The listing builds one solid part. Answer for the finished solid, in the listing's coordinates (mm). Face numbers are marked on the shaded views. A direction names the side the tool comes from. Round coordinates to 2 decimals unless told otherwise and drop trailing zeros. Write each loop counter-clockwise with the first axis right and the second up, starting at its lowest first coordinate (ties: lowest second). Pieces come first, ordered by that corner, then holes. Notation, with made-up numbers: (35.25, 72.25) - (53.25, 72.25) arc R3 ccw to (53.25, 76.25) - close; hole circle Ø2 at (-32.75, 35). An arc over 180 degrees is marked (long way). Use a Markdown table: item, result. Add a question column.
1) A cutting plane is placed at B-B (y = -5). Give the vertices of the cut face in (x, z), then the cut area to 3 significant figures.
2) A tool of negligible diameter and unlimited length cuts with its end or side. For the marked faces 1, 2, 3 and 4, from which of +Z, -Z, +X, -X, +Y, -Y can it reach the whole face along a straight path? Write none if from no direction.
3) A cutting plane is placed at A-A (x = 3). Give the vertices of the cut face in (y, z).
4) Each of these flat-tipped pins is pushed along its axis until it touches: P1, Ø5, axis at x = -3.68, z = 13.02, coming from the -Y side; P2, Ø5, axis at y = -3, z = 27.5, coming from the +X side; P3, Ø3, axis at y = -5, z = 31, coming from the -X side; P4, Ø4, axis at x = -5, z = 22.5, coming from the +Y side. Where does it stop, or does it pass through?
5) Find the intervals of material crossed by probe 1 along Z at (x, y) = (-2.5, 1.5); probe 2 along Z at (x, y) = (-1.5, 7.5); probe 3 along X at (y, z) = (4.75, 11), in increasing order. Write a range as from..to.
6) A cutting plane is placed at D-D (y = 0.5). Give the vertices of the cut face in (x, z), then the cut area to 3 significant figures.
7) Determine the mould class of the marked faces 5, 6 and 7 for opening direction Z: +Z half, -Z half, draft (parallel to the pull), parting line (faces both ways), or undercut.
8) A cutting plane is placed at C-C (x = 0). Give the vertices of the cut face in (y, z).
```python
from build123d import *

# Parameters (mm, degrees)
F1_DEPTH      = 12
F2_SIZE       = 2
F3_R          = 2.5
F4_DEPTH      = 10
F7_DEPTH      = 1
F7_DEPTH_BACK = 1


with BuildPart() as f1:
    # F0 (on Top) → F1 (new body)
    with BuildSketch(Plane.XY):
        Polygon((-9.5, 0), (-4.75, -8.227241), (4.75, -8.227241), (9.5, 0), (4.75, 8.227241), (-4.75, 8.227241), align=None)
    extrude(amount=F1_DEPTH)

    # F2
    f2_edges = [f1.edges().sort_by_distance(p)[0] for p in [
        (-7.125, 4.113621, 0),
        (-7.125, -4.113621, 0),
        (0, -8.227241, 0),
        (7.125, -4.113621, 0),
        (7.125, 4.113621, 0),
        (0, 8.227241, 0),
        (-7.125, 4.113621, 12),
        (-7.125, -4.113621, 12),
        (0, -8.227241, 12),
        (7.125, -4.113621, 12),
        (7.125, 4.113621, 12),
        (0, 8.227241, 12),
    ]]
    chamfer(f2_edges, length=F2_SIZE)

    # F3 (on face) → F4 (join)
    with BuildSketch(Plane.XY.offset(12)):
        Circle(F3_R)
    extrude(amount=F4_DEPTH)

    # F5: F1 across face


with BuildPart() as f1_1:
    add(f1.part)
    add(f1.part.mirror(Plane.XY.offset(22)))

    # F6 (on Front) → F7 (join, two sides)
    with BuildSketch(Plane.XZ) as f7_sk:
        with BuildLine():
            Line((-2.217598, 13.345242), (-2.217598, 15.045078))
            ThreePointArc((-2.217598, 15.045078), (-5.263964, 14.954063), (-5.958645, 11.986564))
            Line((-5.958645, 11.986564), (-4.770151, 11.986564))
            ThreePointArc((-4.770151, 11.986564), (-4.386394, 14.342682), (-2.217598, 13.345242))
        make_face()
    extrude(amount=F7_DEPTH)
    extrude(f7_sk.sketch, amount=-F7_DEPTH_BACK)


solid = f1_1.part
```
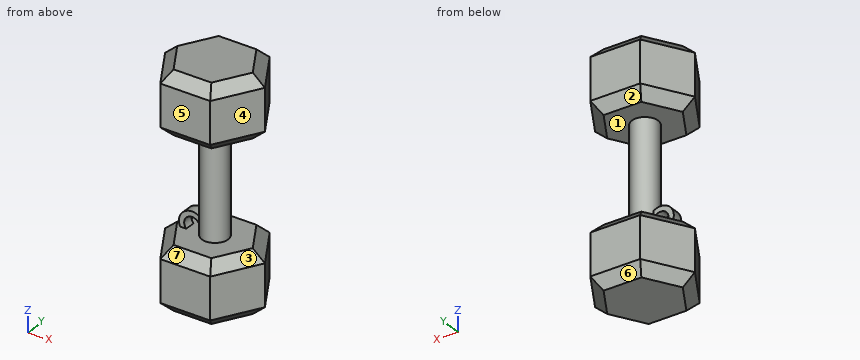
Entries:
| question | item | result |
|---|---|---|
| 1 | outline | (-6.61, 2) - (-4.3, 0) - (4.3, 0) - (6.61, 2) - (6.61, 10) - (4.3, 12) - (-4.3, 12) - (-6.61, 10) - close; (-6.61, 34) - (-4.3, 32) - (4.3, 32) - (6.61, 34) - (6.61, 42) - (4.3, 44) - (-4.3, 44) - (-6.61, 42) - close |
| 1 | area | 299 mm² |
| 2 | face 1 | none |
| 2 | face 2 | +X, -X, +Y |
| 2 | face 3 | +X, -Y |
| 2 | face 4 | +Z, -Z, +X, -Y |
| 3 | outline | (-8.23, 2) - (-6.23, 0) - (6.23, 0) - (8.23, 2) - (8.23, 10) - (6.23, 12) - (-6.23, 12) - (-8.23, 10) - close; (-8.23, 34) - (-6.23, 32) - (6.23, 32) - (8.23, 34) - (8.23, 42) - (6.23, 44) - (-6.23, 44) - (-8.23, 42) - close |
| 4 | P1 | stops at y = -7.71 |
| 4 | P2 | stops at x = 2.45 |
| 4 | P3 | stops at x = -5.09 |
| 4 | P4 | passes through |
| 5 | probe 1 | z = 0..12, 32..44 |
| 5 | probe 2 | z = 1.27..10.73, 33.27..42.73 |
| 5 | probe 3 | x = -5.6..5.6 |
| 6 | outline | (-9.21, 2) - (-6.9, 0) - (6.9, 0) - (9.21, 2) - (9.21, 10) - (6.9, 12) - (2.45, 12) - (2.45, 32) - (6.9, 32) - (9.21, 34) - (9.21, 42) - (6.9, 44) - (-6.9, 44) - (-9.21, 42) - (-9.21, 34) - (-6.9, 32) - (-2.45, 32) - (-2.45, 15.19) arc R2.5 ccw to (-5.96, 12) - (-6.9, 12) - (-9.21, 10) - close; hole (-4.78, 12) - (-2.45, 12) - (-2.45, 13.87) arc R1.5 ccw (long way) to start |
| 6 | area | 527 mm² |
| 7 | face 5 | draft |
| 7 | face 6 | -Z half |
| 7 | face 7 | undercut |
| 8 | outline | (-8.23, 2) - (-6.23, 0) - (6.23, 0) - (8.23, 2) - (8.23, 10) - (6.23, 12) - (2.5, 12) - (2.5, 32) - (6.23, 32) - (8.23, 34) - (8.23, 42) - (6.23, 44) - (-6.23, 44) - (-8.23, 42) - (-8.23, 34) - (-6.23, 32) - (-2.5, 32) - (-2.5, 12) - (-6.23, 12) - (-8.23, 10) - close |
